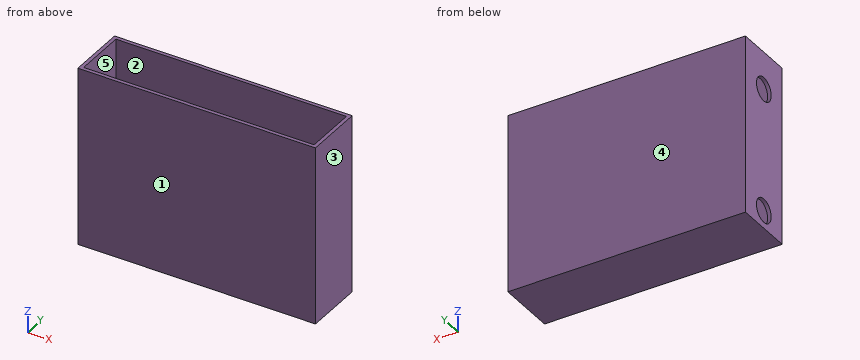
```python
from build123d import *

# Parameters (mm, degrees)
F0_W     = 200
F0_H     = 50
F0_W_2   = 194
F0_H_2   = 44
F1_DEPTH = 150
F2_DEPTH = 5
F3_R     = 10
F4_DEPTH = 25.4
F5_DEPTH = 25.4


with BuildPart() as f1:
    # F0 (on Top) → F1 (new body)
    with BuildSketch(Plane.XY):
        with Locations((1.854228, -17.701853)):
            Rectangle(F0_W, F0_H)
        with Locations((1.854228, -17.701853)):
            Rectangle(F0_W_2, F0_H_2, mode=Mode.SUBTRACT)
    extrude(amount=F1_DEPTH)

    # F0 (on Top) → F2 (join)
    with BuildSketch(Plane.XY):
        with Locations((1.854228, -17.701853)):
            Rectangle(F0_W_2, F0_H_2)
    extrude(amount=F2_DEPTH)

    # F3 (on face) → F4 (cut)
    with BuildSketch(Plane(origin=(-98.145772, 0, 0), x_dir=(0, -1, 0), z_dir=(-1, 0, 0))):
        with Locations((17.701853, 118.406542)):
            Circle(F3_R)
    extrude(amount=-F4_DEPTH, mode=Mode.SUBTRACT)

    # F3 (on face) → F5 (cut)
    with BuildSketch(Plane(origin=(-98.145772, 0, 0), x_dir=(0, -1, 0), z_dir=(-1, 0, 0))):
        with Locations((17.701853, 15)):
            Circle(F3_R)
    extrude(amount=-F5_DEPTH, mode=Mode.SUBTRACT)


solid = f1.part
```
Input: part model. Units: mm. Frame: model coordinates. Face numbers are marked on the shaded views. A direction names the side the tool comes from. Give positions to 0.01 mm unless a question says otherwise; leave off trailing zeros. Write each loop counter-clockwise with the first axis right and the second up, starting at its lowest first coordinate (ties: lowest second). Pieces come first, ordered by that corner, then holes. Notation, with made-up numbers: (44.25, -34.75) - (79.25, -34.75) arc R21 ccw to (79.25, -13.75) - close; hole circle Ø4 at (17.25, 40.25). An arc over 180 degrees is marked (long way). Write item = value, one per line. Start each with the question number.
1) Reachability of the marked faces 1 and 2 from +Z, -Z, +X, -X, +Y, -Y: full face, straight path, thin tool, end or side. Return the list, or none.
2) Cut plane D-D (z = 15). Return loops of the section in (x, y).
3) Cut plane C-C (x = 31.5). Return loops of the section in (y, z), and give its area (3 significant figures).
4) Material intervals for L1, parallel to X at y = -10.5, z = 88; L2, parallel to Y at x = 46.5, z = 93; L3, parallel to Z at x = -49, y = -4, sorted ascending. Write a range as [from, to].
5) Pin query (flat end, axial travel): pin 1 (1.5 mm diameter, centred on x = -7.5, y = -19, fed in from +Z). Return the tip coordinate at first contact, or that it passes through.
6) Cut plane B-B (y = -20). Return loops of the section in (x, z).
7) Draft query along Y for the marked faces 3, 4 and 5. Return one class per face: pulls with the +Y half, pulls with the -Y half, needs draft (parallel to the pull), parting line crosses it, or undercut.
8) Cut plane A-A (z = 135). Return loops of the section in (x, y).
Answers follow:
q1.face_1 = +Z, -Z, +X, -X, -Y
q1.face_2 = +Z
q2.outline = (-98.15, -42.7) - (101.85, -42.7) - (101.85, 7.3) - (-98.15, 7.3) - (-98.15, -7.7) - (-95.15, -7.7) - (-95.15, 4.3) - (98.85, 4.3) - (98.85, -39.7) - (-95.15, -39.7) - (-95.15, -27.7) - (-98.15, -27.7) - close
q3.outline = (-42.7, 0) - (7.3, 0) - (7.3, 150) - (4.3, 150) - (4.3, 5) - (-39.7, 5) - (-39.7, 150) - (-42.7, 150) - close
q3.area = 1,120 mm^2
q4.L1 = [-98.15, -95.15], [98.85, 101.85]
q4.L2 = [-42.7, -39.7], [4.3, 7.3]
q4.L3 = [0, 5]
q5.pin_1 = 5
q6.outline = (-98.15, 0) - (101.85, 0) - (101.85, 150) - (98.85, 150) - (98.85, 5) - (-95.15, 5) - (-95.15, 5.27) - (-98.15, 5.27) - close; (-98.15, 24.73) - (-95.15, 24.73) - (-95.15, 108.67) - (-98.15, 108.67) - close; (-98.15, 128.14) - (-95.15, 128.14) - (-95.15, 150) - (-98.15, 150) - close
q7.face_3 = needs draft
q7.face_4 = pulls with the +Y half
q7.face_5 = undercut
q8.outline = (-98.15, -42.7) - (101.85, -42.7) - (101.85, 7.3) - (-98.15, 7.3) - close; hole (-95.15, -39.7) - (98.85, -39.7) - (98.85, 4.3) - (-95.15, 4.3) - close
